Can you work these out from the model? Positions are in its coordinate system, mm. Face numbers are marked on the shaded views. A direction names the side the tool comes from. Round coordinates to 2 decimals unless told otherwise and drop trailing zeros. Write each loop counter-clockwise with the first axis right and the second up, starting at its lowest first coordinate (ties: lowest second). Pieces come first, ordered by that corner, then holes. Notation, with made-up numbers: (27, 53) -> (61, 53) arc R24 ccw to (61, 84) -> close; hole circle Ø7 at (79.25, 38.25). An arc over 180 degrees is marked (long way). Use CSV: the item, a comma, the result in double quotes.
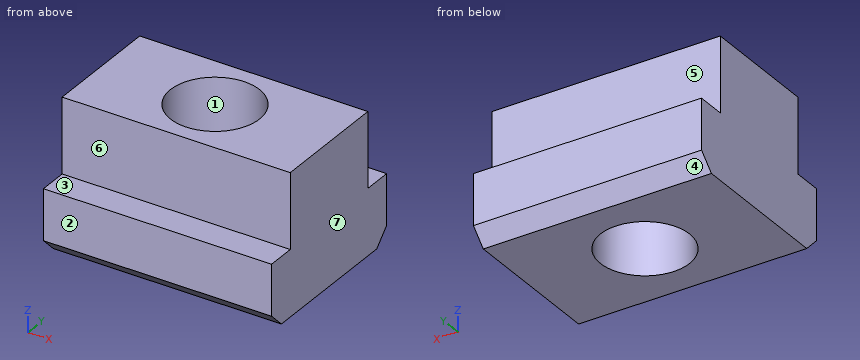
```python
from build123d import *

# Parameters (mm, degrees)
F1_DEPTH = 22.5
F3_D     = 8.8
F4_SIZE  = 1.5


with BuildPart() as f1:
    # F0 (on Right) → F1 (new body)
    with BuildSketch(Plane.YZ):
        Polygon((5.9, 7.4), (-5.9, 7.4), (-5.9, 0), (-8.75, 0), (-8.75, -6.5), (8.75, -6.5), (8.75, 0), (5.9, 0), align=None)
    extrude(amount=-F1_DEPTH)

    # F3 (through all)
    with Locations(Plane.XY.offset(7.4)):
        with Locations((-11.25, 0)):
            Hole(F3_D / 2)

    # F4
    f4_edges = [f1.edges().sort_by_distance(p)[0] for p in [
        (-11.25, -8.75, -6.5),
        (-11.25, 8.75, -6.5),
    ]]
    chamfer(f4_edges, length=F4_SIZE)


solid = f1.part
```
Q1. If we mould it in two halves opening along Y, with no side actions, what happens to the marked faces 1, 2, 3 and 4? For each: released by +Y, released by -Y, zero draft, split by the parting line, or undercut.
Resolved:
face 1,"undercut"
face 2,"released by -Y"
face 3,"zero draft"
face 4,"released by +Y"
Q2. Suppose I cut it at C-C (z = -3). Write out the boundary of the cut face in (x, y).
Resolved:
outline,"(-22.5, -8.75) -> (0, -8.75) -> (0, 8.75) -> (-22.5, 8.75) -> close; hole circle Ø8.8 at (-11.25, 0)"
Q3. Suppose I cut it at A-A (y = 0). Write out the boundary of the cut face in (x, z), and give its area (3 significant figures).
Resolved:
outline,"(-22.5, -6.5) -> (-15.65, -6.5) -> (-15.65, 7.4) -> (-22.5, 7.4) -> close; (-6.85, -6.5) -> (0, -6.5) -> (0, 7.4) -> (-6.85, 7.4) -> close"
area,"190 mm^2"
Q4. On a 3-axis mill with a long thin cutter (end or side, diameter ignored), from which of +Z, -Z, +X, -X, +Y, -Y can I reach the whole of each face in a straight line? I mean the marked faces 5, 6 and 7. Say none if no direction works.
Resolved:
face 5,"+Z, +X, -X, +Y"
face 6,"+Z, +X, -X, -Y"
face 7,"+Z, -Z, +X, +Y, -Y"
Q5. Suppose I cut it at D-D (x = -5.75). Write out the boundary of the cut face in (y, z), and give its area (3 significant figures).
Resolved:
outline,"(-8.75, -5) -> (-7.25, -6.5) -> (7.25, -6.5) -> (8.75, -5) -> (8.75, 0) -> (5.9, 0) -> (5.9, 7.4) -> (-5.9, 7.4) -> (-5.9, 0) -> (-8.75, 0) -> close"
area,"199 mm^2"
Q6. Will these pins go through, and if not, where does the flat tip stop? P1, Ø3.5, axis at x = -7.5, z = 5, coming from the +Y side; P2, Ø5.5, axis at x = -11.25, y = 0, coming from the +Z side; P3, Ø1.4, axis at x = -6, y = 8, coming from the +Z side; P4, Ø8, axis at x = -14, z = 5, coming from the -Y side.
Resolved:
P1,"stops at y = 5.9"
P2,"passes through"
P3,"stops at z = 0"
P4,"stops at y = -5.9"
Q7. Suppose I cut it at B-B (x = -11.25). Write out the boundary of the cut face in (y, z).
Resolved:
outline,"(-8.75, -5) -> (-7.25, -6.5) -> (-4.4, -6.5) -> (-4.4, 7.4) -> (-5.9, 7.4) -> (-5.9, 0) -> (-8.75, 0) -> close; (4.4, -6.5) -> (7.25, -6.5) -> (8.75, -5) -> (8.75, 0) -> (5.9, 0) -> (5.9, 7.4) -> (4.4, 7.4) -> close"
Q8. Please list where these lines run through material, in increasing order: probe 1 along Y at (x, z) = (-11.25, -1.25); probe 2 along Y at (x, z) = (-11.25, 4.5); probe 3 along Y at (x, z) = (-1.5, 2).
Resolved:
probe 1,"y = -8.75 to -4.4, 4.4 to 8.75"
probe 2,"y = -5.9 to -4.4, 4.4 to 5.9"
probe 3,"y = -5.9 to 5.9"
